from build123d import *

# Parameters (mm, degrees)
PAD030_DEPTH    = 1
SKETCH049_W     = 8.1
SKETCH049_H     = 3.05
POCKET019_DEPTH = 0.5
POCKET020_DEPTH = 0.25
POCKET021_DEPTH = 0.25
CHAMFER008_SIZE = 0.25
SKETCH052_W     = 3
SKETCH052_H     = 8
PAD031_DEPTH    = 0.5
SKETCH053_R     = 3
SKETCH053_R_2   = 1.3
PAD032_DEPTH    = 3.5


with BuildPart() as part:
    # Sketch048 (on Face2 of Binder014) → Pad030 (new body)
    with BuildSketch(Plane(origin=(0, 0, -13), x_dir=(1, 0, 0), z_dir=(0, 0, -1))):
        Polygon((129, -5.333333), (129, 44.999997), (118.3, 44.999997), (118.3, 47.899997), (103.4, 47.899997), (103.4, 44.999997), (91.3, 44.999997), (91.3, 47.899997), (76.4, 47.899997), (76.4, 44.999997), (65.65, 44.999997), (65.65, 7.016667), (78, -5.333333), align=None)
    extrude(amount=-PAD030_DEPTH)

    # Sketch049 (on Face14 of Pad030) → Pocket019 (cut)
    with BuildSketch(Plane(origin=(0, 0, -13), x_dir=(1, 0, 0), z_dir=(0, 0, -1))):
        with Locations((92, -3.808333)):
            Rectangle(SKETCH049_W, SKETCH049_H)
        with Locations((115, -3.808333)):
            Rectangle(SKETCH049_W, SKETCH049_H)
    extrude(amount=-POCKET019_DEPTH, mode=Mode.SUBTRACT)

    # Sketch050 (on Face5 of Pocket019) → Pocket020 (cut)
    with BuildSketch(Plane.XY.offset(-12)):
        Polygon((78, 5.333333), (78.7071067812, 5.333333), (66.15, -7.2237737812), (66.15, -44.999997), (65.65, -44.999997), (65.65, -7.016667), align=None)
    extrude(amount=-POCKET020_DEPTH, mode=Mode.SUBTRACT)

    # Sketch051 (on Face5 of Pocket020) → Pocket021 (cut)
    with BuildSketch(Plane.XY.offset(-12)):
        Polygon((66.15, -14.649997), (101.3571067812, -14.649997), (111.2071067812, -24.499997), (129, -24.499997), (129, -24.999997), (111, -24.999997), (101.15, -15.149997), (66.15, -15.149997), align=None)
    extrude(amount=-POCKET021_DEPTH, mode=Mode.SUBTRACT)

    # Chamfer008
    chamfer008_edges = [part.edges().sort_by_distance(p)[0] for p in [
        (129, -9.583332, -12),
        (129, -34.999997, -12),
    ]]
    chamfer(chamfer008_edges, length=CHAMFER008_SIZE)

    # Sketch052 (on Face4 of Chamfer008) → Pad031 (join)
    with BuildSketch(Plane(origin=(0, 0, -13), x_dir=(1, 0, 0), z_dir=(0, 0, -1))):
        Polygon((66.0035533906, 6.6631136094), (71.6604076401, 1.0062593599), (69.5390872965, -1.1150609836), (63.882233047, 4.5417932658), align=None)
        with Locations((64.15, 16.016667)):
            Rectangle(SKETCH052_W, SKETCH052_H)
        with Locations((64.15, 35.999997)):
            Rectangle(SKETCH052_W, SKETCH052_H)
    extrude(amount=-PAD031_DEPTH)

    # Sketch053 (on Face7 of Pad031) → Pad032 (join)
    with BuildSketch(Plane.XY.offset(-12)):
        with Locations((77.7, -18.249997)):
            Circle(SKETCH053_R)
        with Locations((77.7, -18.249997)):
            Circle(SKETCH053_R_2, mode=Mode.SUBTRACT)
        with Locations((93.3, -18.249997)):
            Circle(SKETCH053_R)
        with Locations((93.3, -18.249997)):
            Circle(SKETCH053_R_2, mode=Mode.SUBTRACT)
    extrude(amount=PAD032_DEPTH)


solid = part.part
Source: CAD feature listing. Evaluate the final solid. Frame: model axes, mm. A direction names the side the tool comes from. Give positions to 0.01 mm unless a question says otherwise; leave off trailing zeros. Order: outer loops, then holes, each group sorted by start corner. A loop starts at its lowest first (then second) coordinate and runs counter-clockwise, first axis right, second up. Notation, with made-up numbers: (71, -19.5) -> (102, -19.5) arc R30 ccw to (102, 10.5) -> close; hole circle Ø10 at (58.25, 8.5). An arc over 180 degrees is marked (long way). Write item = value, one per line.
Q1. Cut plane B-B, the plane z = -10.55. Output: boundary loops of the cut face in (x, y), and give its area (3 significant figures).
Data:
outline = circle Ø6 at (77.7, -18.25); circle Ø6 at (93.3, -18.25); hole circle Ø2.6 at (77.7, -18.25); hole circle Ø2.6 at (93.3, -18.25)
area = 45.9 mm^2
Q2. Cut plane A-A, the plane x = 93.3. Output: boundary loops of the cut face in (y, z).
Data:
outline = (-45, -13) -> (2.28, -13) -> (2.28, -12.5) -> (5.33, -12.5) -> (5.33, -12) -> (-14.65, -12) -> (-14.65, -12.25) -> (-15.15, -12.25) -> (-15.15, -12) -> (-15.25, -12) -> (-15.25, -8.5) -> (-16.95, -8.5) -> (-16.95, -12) -> (-19.55, -12) -> (-19.55, -8.5) -> (-21.25, -8.5) -> (-21.25, -12) -> (-45, -12) -> close
Q3. Cut plane D-D, the plane x = 100. Output: boundary loops of the cut face in (y, z).
Data:
outline = (-45, -13) -> (5.33, -13) -> (5.33, -12) -> (-14.65, -12) -> (-14.65, -12.25) -> (-15.15, -12.25) -> (-15.15, -12) -> (-45, -12) -> close
Q4. Pull-direction query (Y, two-part tool) for faces 4 (the face through (96.07, -19.4, -10.27)), 5 (the face through (68, -3, -12.5)), 6 (the face through (93.999, -17.154, -10.274)); classes: released by +Y, released by -Y, zero draft, split by the parting line, or undercut.
Data:
face_4 = split by the parting line
face_5 = zero draft
face_6 = undercut
Q5. Set-up query: faces 1 (the face through (92, 4, -12.5)), 2 (the face through (64, -16, -12.5)), 3 (the face through (75.319, -20.075, -10.274)). Return all of +Z, -Z, +X, -X, +Y, -Y with unobstructed straight access to the full face (end or side cutting, diameter ignored); none if empty.
Data:
face_1 = -Z, +Y
face_2 = +Z, -X, +Y, -Y
face_3 = +Z
Q6. Cut plane C-C, the plane x = 112. Output: boundary loops of the cut face in (y, z).
Data:
outline = (-47.9, -13) -> (2.28, -13) -> (2.28, -12.5) -> (5.33, -12.5) -> (5.33, -12) -> (-24.5, -12) -> (-24.5, -12.25) -> (-25, -12.25) -> (-25, -12) -> (-47.9, -12) -> close
Q7. Material intervals for line 1 (Y direction, x = 93.3, z = -9.55); line 2 (Z direction, x = 119, y = -35.5); line 3 (X direction, y = -36.5, z = -12.35), sorted ascending. Write a range as from..to.
Data:
line_1 = -21.25..-19.55, -16.95..-15.25
line_2 = -13..-12
line_3 = 65.65..129
Q8. Pin query (flat end, axial travel): pin 1 (1.1 mm diameter, centred on y = -46.5, z = -12.5, fed in from -X); pin 2 (5 mm diameter, centred on x = 70.5, y = -25, fed in from +Z); pin 3 (1 mm diameter, centred on y = -23, z = -12.5, fed in from -X). Return the tip coordinate at first contact, or that it passes through.
Data:
pin_1 = 76.4
pin_2 = -12
pin_3 = 65.65
